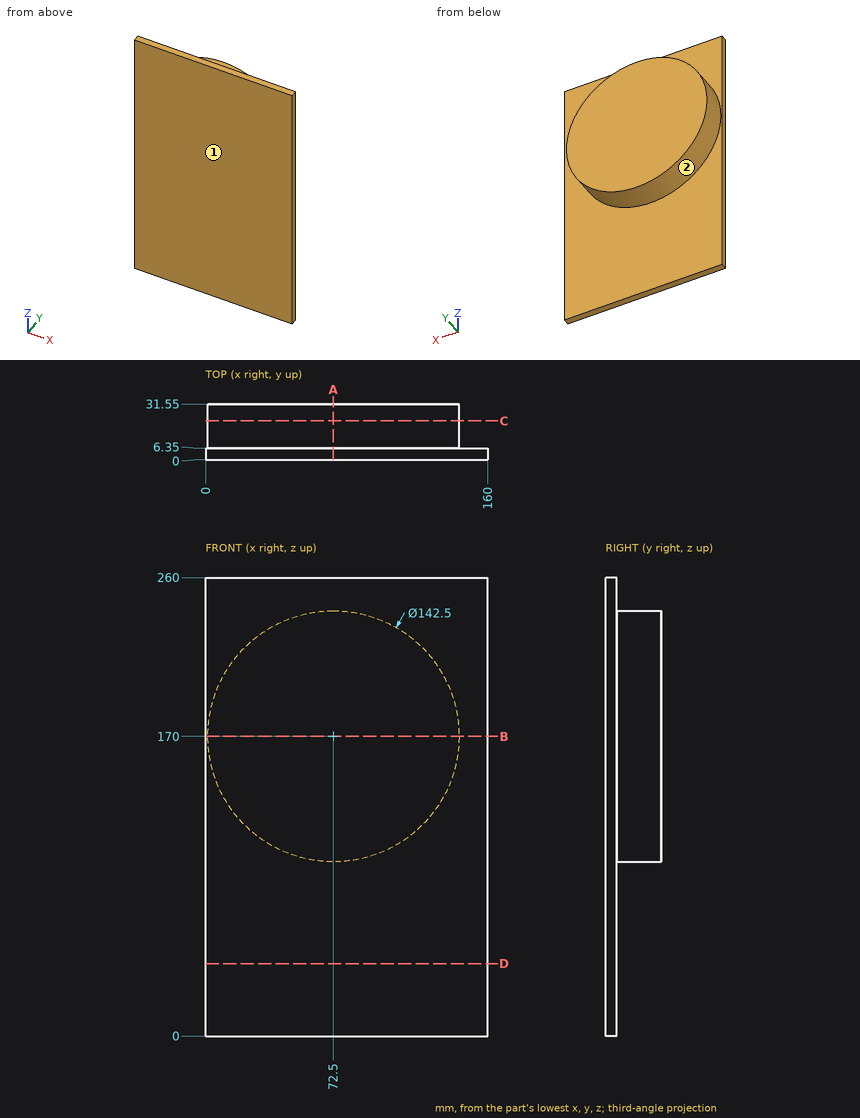
Drawing for the job (mm, zero at the part's lowest x, y, z). A direction names the side the tool comes from. Coordinates: 2 decimals unless noted, no trailing zeros. Order: outer loops, then holes, each group sorted by start corner. A loop starts at its lowest first (then second) coordinate and runs counter-clockwise, first axis right, second up. Notation, with made-up numbers: (24, 68.25) - (65, 68.25) arc R17 ccw to (65, 83.25) - close; hole circle Ø2 at (-21, 22.5). An arc over 180 degrees is marked (long way). Use a Markdown table: item, result. Add a question column.
(1) Saw through at A-A (x = 72.5). Give the cut face in (y, z).
(2) Saw through at C-C (y = 22). Give the cut face in (x, z), then the cut area to 3 significant figures.
(3) Saw through at B-B (z = 170). Give the cut face in (x, y), then the cut area to 3 significant figures.
(4) Flat gauge pins, fed straight in: pin 1 (3 mm diameter, centred on x = 129, y = 15, fed in from -Z); pin 2 (10 mm diameter, centred on x = 78, y = 17, fed in from +Z); pin 3 (6 mm diameter, centred on x = 34, y = 16.5, fed in from -Z). Where does each tip first touch, or does it go through?
(5) Saw through at D-D (z = 41). Give the cut face in (x, y), then the cut area to 3 significant figures.
(6) Which spindle directions (+Z, -Z, +X, -X, +Y, -Y) get a long thin tool onto all of the face, cutting with end or side? Do the marked faces 1 and 2. Say none if no direction does.
(7) Drill centre lines: line 1 along Y through (x, z) = (119, 39.5); line 2 along X through (y, z) = (27, 123.5); line 3 along X through (y, z) = (26.5, 204.5). Where is each one in solid material? Low to high. Write a range as [from, to].
Solved:
| question | item | result |
|---|---|---|
| 1 | outline | (0, 0) - (6.35, 0) - (6.35, 98.75) - (31.55, 98.75) - (31.55, 241.25) - (6.35, 241.25) - (6.35, 260) - (0, 260) - close |
| 2 | outline | circle Ø142.5 at (72.5, 170) |
| 2 | area | 15,900 mm² |
| 3 | outline | (0, 0) - (160, 0) - (160, 6.35) - (143.75, 6.35) - (143.75, 31.55) - (1.25, 31.55) - (1.25, 6.35) - (0, 6.35) - close |
| 3 | area | 4,610 mm² |
| 4 | pin 1 | stops at z = 124.71 |
| 4 | pin 2 | stops at z = 241.25 |
| 4 | pin 3 | stops at z = 108.22 |
| 5 | outline | (0, 0) - (160, 0) - (160, 6.35) - (0, 6.35) - close |
| 5 | area | 1,020 mm² |
| 6 | face 1 | +Z, -Z, +X, -X, -Y |
| 6 | face 2 | +Y |
| 7 | line 1 | y = [0, 6.35] |
| 7 | line 2 | x = [18.52, 126.48] |
| 7 | line 3 | x = [10.16, 134.84] |
